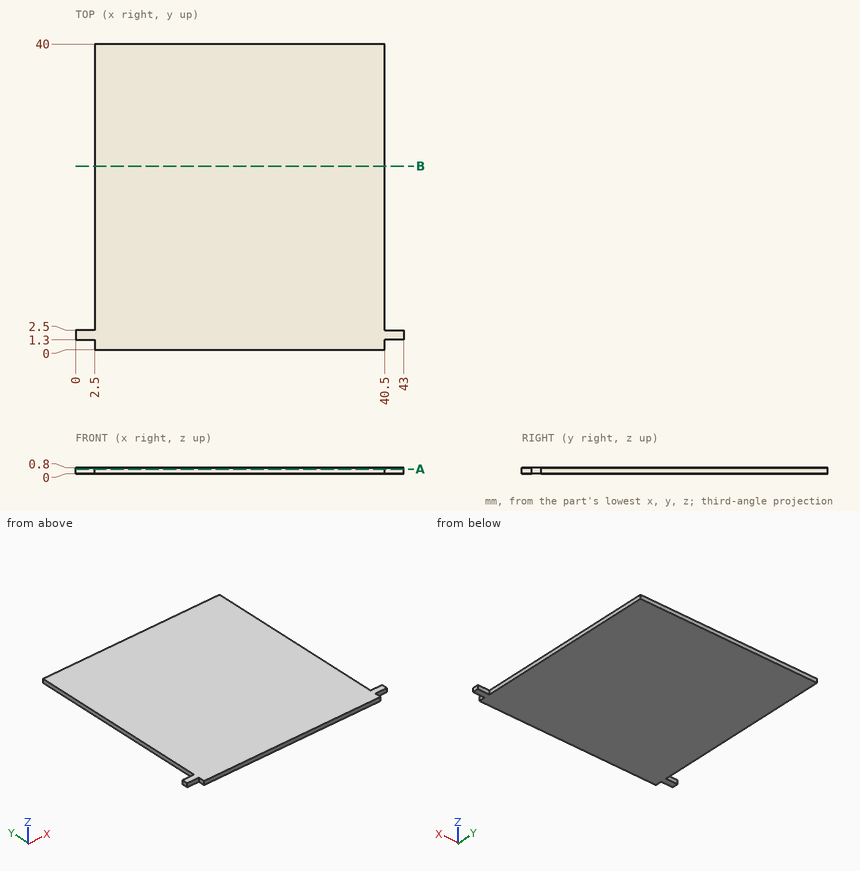
Job drawing, mm, ordinate dimensions from the low corner. One solid piece. Coordinates: 2 decimals unless noted, no trailing zeros. Write each loop counter-clockwise with the first axis right and the second up, starting at its lowest first coordinate (ties: lowest second). Pieces come first, ordered by that corner, then holes. Notation, with made-up numbers: M -33,-21.75 L 1,-21.75 A28 ccw 1,15.25 Z; hole C 7.5,-6.75 d10. An arc over 180 degrees is marked long. Answer as a JSON object with one key per item and string values. Group by question number.
1) Pin check, flat tip, straight feed: pin 1 Ø4 at (x, y) = (14.5, 16.5) entering from -Z. Stop position of the tip, or through.
2) Saw through at B-B (y = 24). Write the cut outline in (x, z), plus the area to 3 significant figures.
3) Saw through at A-A (z = 0.6). Write the cut outline in (x, y), plus the area to 3 significant figures.
4) Wall check: line 1 (X direction, y = 27, z = 0.4); line 2 (Y direction, x = 2, z = 0.15). Give the ranges that are in metal, low to high. Write a range as from..to.
Values follow:
{
 "1": {"pin 1": "stops at z = 0"},
 "2": {"outline": "M 2.5,0 L 40.5,0 L 40.5,0.8 L 2.5,0.8 Z", "area": "30.4 mm2"},
 "3": {"outline": "M 0,1.3 L 2.5,1.3 L 2.5,0 L 40.5,0 L 40.5,1.3 L 43,1.3 L 43,2.5 L 40.5,2.5 L 40.5,40 L 2.5,40 L 2.5,2.5 L 0,2.5 Z", "area": "1,530 mm2"},
 "4": {"line 1": "x = 2.5..40.5", "line 2": "y = 1.3..2.5"}
}
